Part model, mm, in its own coordinate system. A direction names the side the tool comes from. Coordinates: 2 decimals unless noted, no trailing zeros. Write each loop counter-clockwise with the first axis right and the second up, starting at its lowest first coordinate (ties: lowest second). Pieces come first, ordered by that corner, then holes. Notation, with made-up numbers: (88, 60) -> (113, 60) arc R28 cw to (113, 79) -> close; hole circle Ø8 at (-10.5, 52). An arc over 180 degrees is marked (long way). Write item = value, one per line. Start each with the question number.
Q1. Band-saw the part on C-C, the plane z = 16.75. List the corners of the cut face in (x, y).
Q2. Band-saw the part on D-D, the plane x = -3. List the corners of the cut face in (y, z), plus the area to 3 significant figures.
Q3. Probe line 1 (Y direction, x = 0, z = 9); line 2 (X direction, y = 7.25, z = 23); line 3 (Y direction, x = -2, z = 6.25). List the from-to ranges inside material, lowest first.
Q4. Band-saw the part on A-A, the plane y = 8. List the corners of the cut face in (x, z), plus the area to 3 significant figures.
Q5. Pull direction Y, two halves, no side cores. Call faces 5 (the cylindrical face through (0.954, -2.229, 14.79)), 6 (the cylindrical face through (-5.713, 5.752, 2.465)), 7 (the cylindrical face through (0, -10, 15)), 8 (the flat face through (10, 4, 15)): released by +Y, released by -Y, zero draft, split by the parting line, or undercut.
Q6. Tool access for faces 1 (the flat face through (-7, 8, 5)), 2 (the flat face through (9, 5, 2)), 3 (the flat face through (3, -9, 5)), 4 (the flat face through (-5, 3, 26)): list every direction of +Z, -Z, +X, -X, +Y, -Y with a clear straight run to the whole face (end or side of a thin tool).
Q7. Band-saw the part on B-B, the plane x = 0. List the corners of the cut face in (y, z), plus the area to 3 significant figures.
Q8. Pin check, flat tips, straight feed: P1, Ø1.5, axis at x = 3.5, y = -7, coming from the +Z side; P2, Ø2, axis at y = 9, z = 3.5, coming from the +X side; P3, Ø3.5, axis at x = 5, z = 27.5, coming from the -Y side. Stop position of each tip, or through.
Autodesk Inventor part; units mm, degrees
ref_plane "YZ Plane" through (0, 0, 0) normal (1, 0, 0) x (0, 1, 0)
ref_plane "XZ Plane" through (0, 0, 0) normal (0, 1, 0) x (-1, 0, 0)
ref_plane "XY Plane" through (0, 0, 0) normal (0, 0, 1) x (1, 0, 0)
sketch "Finger Body" plane through (0, 0, 0) normal (0, 0, 1) x (1, 0, 0)
  line L0 (-10, 10) -> (10, 10)
  line L1 (10, 10) -> (10, -10)
  line L2 (10, -10) -> (-10, -10)
  line L3 (-10, -10) -> (-10, 10)
  arc A0 (-10, 0) -> (10, 0) centre (0, 0) ccw
  line L4 (-10, 0) -> (10, 0)
  circle A1 centre (-7.5, 7.5) radius 2.5
  circle A2 centre (7.5, 7.5) radius 2.5
  circle A3 centre (0, 0) radius 8.75
  line L5 (0, -8.75) -> (1, -8.75) construction
  line L6 (1, 8.6927) -> (1, -8.75)
  line L7 (-1, 8.6927) -> (-1, -8.6927)
  line L8 (-1, -9.9499) -> (-1, -10)
  circle A4 centre (0, 7.25) radius 1.5
  circle A5 centre (0, -1.929) radius 1
  point P0 (1, -8.6927)
  point P1 (10, 7.5)
  point P2 (7.5, 10)
  point P3 (-7.5, 10)
  point P4 (-10, 7.5)
  dimension "d0" = 20
  dimension "d1" = 20
  dimension "d2" = 10
  dimension "d3" = 10
  dimension "d4" = 5
  dimension "d5" = 2.5
  dimension "d6" = 2.5
  dimension "d7" = 5
  dimension "d8" = 2.5
  dimension "d9" = 2.5
  dimension "d10" = 17.5
  dimension "d42" = 3
  dimension "d43" = 0
  dimension "d44" = 0
  dimension "d45" = 9.179
  dimension "d46" = 0
sketch "Cap Imprint (DNE)" plane through (0, 0, 0) normal (0, 0, 1) x (1, 0, 0)
  circle A0 centre (0, 0) radius 8.75
  arc A1 (-10, 0) -> (10, 0) centre (0, 0) ccw
  line L0 (-10, -10) -> (-10, 10)
  line L1 (-10, 10) -> (10, 10)
  line L2 (10, 10) -> (10, -10)
  line L3 (1, 8.6927) -> (1, -8.75)
  line L4 (-1, 8.6927) -> (-1, -8.6927)
  circle A2 centre (-7.5, 7.5) radius 2.5
  circle A3 centre (7.5, 7.5) radius 2.5
  circle A4 centre (0, 0) radius 0.5
  dimension "d15" = 1
extrude "FingerLength (Scale for each finger)" add sketch "Finger Body" along normal blind 30 contours L0 A2 A3 A1 | A1 A3 | A1 A3 L4 L3 | A2 A3 | L4 A3 A0 | A3 A1 | A1 A3 L7 A4 L4 | L1 L4 A3 A2 | A3 A2 | A2 A3 L4 L6 A4 | L4 L7 A3 | L6 A4 A3 | A3 A4 L7 | L7 A4 L6 L4 | L4 L6 A5 L7 | L7 A5 L6 A3 | A3 L6 L4
sketch "Sketch3" plane through (0, 0, 30) normal (0, 0, 1) x (1, 0, 0)
  arc A0 (-7.5, 10) -> (-10, 7.5) centre (-7.5, 7.5) ccw
  line L0 (-10, 7.5) -> (-7, 7.5)
  line L1 (-7, 7.5) -> (-6.5, 7.5)
  line L2 (-6.5, 7.5) -> (-3.5, 7.5)
  line L3 (-3.5, 7.5) -> (-3, 7.5)
  arc A1 (10, 7.5) -> (7.5, 10) centre (7.5, 7.5) ccw
  line L4 (10, 7.5) -> (7, 7.5)
  line L5 (7, 7.5) -> (6.5, 7.5)
  line L6 (6.5, 7.5) -> (3.5, 7.5)
  line L7 (3.5, 7.5) -> (3, 7.5)
  line L8 (-6.5, 7.5) -> (-3.5, 7.5)
  line L9 (-3.5, 7.5) -> (-3.5, -2.5)
  line L10 (-3.5, -2.5) -> (-6.5, -2.5)
  line L11 (-6.5, -2.5) -> (-6.5, 7.5)
  line L12 (6.5, 7.5) -> (3.5, 7.5)
  line L13 (3.5, 7.5) -> (3.5, -2.5)
  line L14 (3.5, -2.5) -> (6.5, -2.5)
  line L15 (6.5, -2.5) -> (6.5, 7.5)
  line L16 (-6.5, 2.5) -> (6.5, 2.5)
  line L17 (-6.5, 3.5) -> (6.5, 3.5)
  line L18 (-6.5, 1.5) -> (6.5, 1.5)
  point P0 (0, 0)
  point P1 (-3.5, 1.5)
  point P2 (-3.5, 3.5)
  point P3 (3.5, 1.5)
  point P4 (3.5, 3.5)
  dimension "d18" = 3
  dimension "d19" = 0.5
  dimension "d20" = 3
  dimension "d21" = 0.5
  dimension "d22" = 3
  dimension "d23" = 0.5
  dimension "d24" = 3
  dimension "d25" = 0.5
  dimension "d26" = 10
  dimension "d27" = 10
  dimension "d28" = 1
  dimension "d29" = 1
extrude "Extrusion2" cut sketch "Sketch3" against normal blind 4 contours L17 L9 L16 L11 | L16 L9 L18 L11 | L17 L15 L16 L13 | L16 L15 L18 L13
sketch "Sketch4" plane through (10, 0, 0) normal (1, 0, 0) x (0, 0, -1)
  line L0 (0, -10) -> (-30, -10)
  line L1 (-30, 0) -> (-30, -10)
  line L2 (-30, 0) -> (-30, 7.5)
  line L3 (-30, 10) -> (-30, 7.5)
  line L4 (0, 10) -> (-30, 10)
  line L5 (0, 0) -> (0, 7.5)
  line L6 (0, 10) -> (0, 7.5)
  line L7 (0, 0) -> (0, -10)
  line L8 (0, 7.5) -> (-30, 7.5)
  line L9 (-30, 7.5) -> (-30, -2.5)
  line L10 (-30, -8.6927) -> (-30, 8.6927)
  line L11 (-30, -2.5) -> (-22.5, -10)
  dimension "d32" = 10
  dimension "d33" = 135
extrude "Extrusion3" cut sketch "Sketch4" against normal up to surface (20 mm away) contours L0 L1 L11
sketch "Sketch5" plane through (0, 0, 0) normal (0, 0, -1) x (-1, 0, 0)
  arc A0 (-7.5, 10) -> (-10, 7.5) centre (-7.5, 7.5) ccw
  line L0 (-10, 0) -> (-10, 7.5)
  arc A1 (-10, 0) -> (10, 0) centre (0, 0) ccw
  line L1 (10, 7.5) -> (10, 0)
  arc A2 (10, 7.5) -> (7.5, 10) centre (7.5, 7.5) ccw
  line L2 (-7.5, 10) -> (7.5, 10)
  circle A3 centre (-7.5, 7.5) radius 2.5
  circle A4 centre (7.5, 7.5) radius 2.5
  line L3 (-7.5, 5) -> (-10, 5)
  line L4 (-10, 0) -> (-10, 7.5)
  line L5 (7.5, 5) -> (10, 5)
  line L6 (-5, 7.5) -> (-5, 10)
  line L7 (5, 7.5) -> (5, 10)
  line L8 (-1, -8.6927) -> (-1, -9.9499)
  line L9 (1, -8.6927) -> (1, -9.9499)
  line L10 (-2, -8.6927) -> (-2, -9.9499)
  line L11 (-3.5, -8.6927) -> (-3.5, -9.9499)
  line L12 (2, -8.6927) -> (2, -9.9499)
  line L13 (3.5, -8.6927) -> (3.5, -9.9499)
  line L14 (-3.5, -8.6927) -> (-2, -8.6927)
  line L15 (2, -8.6927) -> (3.5, -8.6927)
  point P0 (2, -9.798)
  point P1 (3.5, -9.3675)
  point P2 (-3.5, -9.3675)
  point P3 (-2, -9.798)
  dimension "d38" = 1
  dimension "d39" = 1.5
  dimension "d40" = 1
  dimension "d41" = 1.5
extrude "Extrusion4" cut sketch "Sketch5" against normal blind 5 contours A3 A0 | L2 L6 A3 | A3 L3 L0 | L2 A4 L7 | A2 A4 | L11 L14 L10 A1 | L1 L5 A4 | A1 L12 L15 L13
sketch "End Imprint (DNE)" plane through (0, 0, 0) normal (0, 0, -1) x (-1, 0, 0)
  line L0 (-5, 10) -> (-5, 7.5)
  arc A0 (-7.5, 5) -> (-5, 7.5) centre (-7.5, 7.5) ccw
  line L1 (-7.5, 5) -> (-10, 5)
  line L2 (-10, 0) -> (-10, 5)
  arc A1 (-10, 0) -> (-3.5, -9.3675) centre (0, 0) ccw
  line L3 (-3.5, -9.3675) -> (-3.5, -8.6927)
  line L4 (-3.5, -8.6927) -> (-2, -8.6927)
  line L5 (-2, -8.6927) -> (-2, -9.798)
  arc A2 (-2, -9.798) -> (2, -9.798) centre (0, 0) ccw
  line L6 (2, -9.798) -> (2, -8.6927)
  line L7 (2, -8.6927) -> (3.5, -8.6927)
  line L8 (3.5, -8.6927) -> (3.5, -9.3675)
  arc A3 (3.5, -9.3675) -> (10, 0) centre (0, 0) ccw
  line L9 (10, 5) -> (10, 0)
  line L10 (10, 5) -> (7.5, 5)
  arc A4 (5, 7.5) -> (7.5, 5) centre (7.5, 7.5) ccw
  line L11 (5, 7.5) -> (5, 10)
  line L12 (-5, 10) -> (5, 10)
  arc A5 (-7.5, 5) -> (-5, 7.5) centre (-7.5, 7.5) ccw
  line L13 (-5, 10) -> (-5, 7.5)
  line L14 (-7.5, 10) -> (-5, 10)
  arc A6 (-7.5, 10) -> (-10, 7.5) centre (-7.5, 7.5) ccw
  line L15 (-10, 5) -> (-10, 7.5)
  line L16 (-7.5, 5) -> (-10, 5)
  arc A7 (10, 7.5) -> (7.5, 10) centre (7.5, 7.5) ccw
  line L17 (5, 10) -> (7.5, 10)
  line L18 (5, 7.5) -> (5, 10)
  arc A8 (5, 7.5) -> (7.5, 5) centre (7.5, 7.5) ccw
  line L19 (10, 5) -> (7.5, 5)
  line L20 (10, 7.5) -> (10, 5)
  line L21 (2, -9.798) -> (2, -8.6927)
  arc A9 (2, -9.798) -> (3.5, -9.3675) centre (0, 0) ccw
  line L22 (3.5, -8.6927) -> (3.5, -9.3675)
  line L23 (2, -8.6927) -> (3.5, -8.6927)
  line L24 (-3.5, -9.3675) -> (-3.5, -8.6927)
  arc A10 (-3.5, -9.3675) -> (-2, -9.798) centre (0, 0) ccw
  line L25 (-2, -8.6927) -> (-2, -9.798)
  line L26 (-3.5, -8.6927) -> (-2, -8.6927)
properties part number "Fingertip Midpart"
Ans:
q1.outline = (-10, 0) arc R10 ccw to (10, 0) -> (10, 7.5) arc R2.5 ccw to (7.5, 10) -> (-7.5, 10) arc R2.5 ccw to (-10, 7.5) -> close; hole circle Ø3 at (0, 7.25); hole circle Ø2 at (0, -1.93)
q2.outline = (-9.54, 5) -> (-8.69, 5) -> (-8.69, 0) -> (10, 0) -> (10, 30) -> (-2.5, 30) -> (-9.54, 22.96) -> close
q2.area = 557 mm2
q3.line_1 = -10 to -2.93, -0.93 to 5.75, 8.75 to 10
q3.line_2 = -10 to -1.5, 1.5 to 10
q3.line_3 = -9.8 to 10
q4.outline = (-9.95, 5) -> (-5, 5) -> (-5, 0) -> (-1.3, 0) -> (-1.3, 30) -> (-9.95, 30) -> close; (1.3, 0) -> (5, 0) -> (5, 5) -> (9.95, 5) -> (9.95, 30) -> (1.3, 30) -> close
q4.area = 470 mm2
q5.face_5 = undercut
q5.face_6 = released by +Y
q5.face_7 = released by -Y
q5.face_8 = zero draft
q6.face_1 = -Z, -X, +Y
q6.face_2 = -Z, +X, +Y
q6.face_3 = -Z, -Y
q6.face_4 = +Z
q7.outline = (-10, 0) -> (-2.93, 0) -> (-2.93, 29.57) -> (-10, 22.5) -> close; (-0.93, 0) -> (5.75, 0) -> (5.75, 30) -> (-0.93, 30) -> close; (8.75, 0) -> (10, 0) -> (10, 30) -> (8.75, 30) -> close
q7.area = 422 mm2
q8.P1 = 26.25
q8.P2 = 5
q8.P3 = -6.75
